The model under review builds one solid part; all positions refer to its coordinate system, in mm. Round coordinates to 2 decimals unless told otherwise and drop trailing zeros. Order: outer loops, then holes, each group sorted by start corner. A loop starts at its lowest first (then second) coordinate and runs counter-clockwise, first axis right, second up. Notation, with made-up numbers: (38, -6.5) -> (85, -6.5) arc R18 cw to (85, 21.5) -> close; hole circle Ø1 at (61, -32). An arc over 180 degrees is marked (long way). Return JSON: item names as keys, results as strings. Group by question number.
from build123d import *

# Parameters (mm, degrees)
BOSS_EXTRUDE1_DEPTH = 6.35
SKETCH2_R           = 12.5
CUT_EXTRUDE1_DEPTH  = 414.4708728


with BuildPart() as part:
    # Sketch1 → Boss-Extrude1 (new body)
    with BuildSketch(Plane.XY):
        Polygon((-381.094249826, -159.734501203), (-381.094249826, 25), (380.905750174, 25), (380.905750174, -160.265445134), align=None)
    extrude(amount=BOSS_EXTRUDE1_DEPTH)

    # Sketch2 → Cut-Extrude1 (cut, through all)
    with BuildSketch(Plane.XY.offset(6.35)):
        Circle(SKETCH2_R)
    extrude(amount=-CUT_EXTRUDE1_DEPTH, mode=Mode.SUBTRACT)


solid = part.part
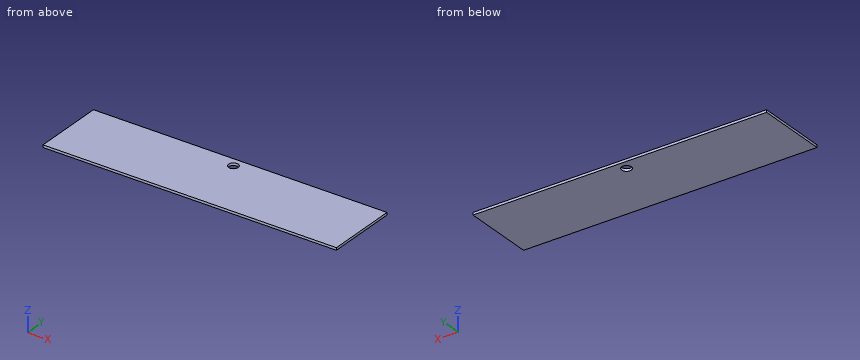
Item 1: Insertion check: pin 1 Ø3 at (x, z) = (264, 4) entering from -Y; pin 2 Ø1.5 at (x, z) = (-146.5, 1) entering from -Y. Each pin has a flat end and moves straight along its axis. Give the tip position at first contact, or say it passes through.
Item 2: Consider section B-B on y = 0. State the section outline as (x, z) points.
Item 3: Wall thickness on line 1 along Y through (x, z) = (237, 2.75); line 2 along Y through (x, z) = (-193.5, 0.5); line 3 along Y through (x, z) = (0, 1.5): over which ranges is each line inside the solid? List them lowest first.
Item 4: Consider section A-A on x = -3. State the section outline as (y, z) points.
Values:
{
 "1": {"pin 1": "y = -160.19", "pin 2": "y = -159.9"},
 "2": {"outline": "(-381.09, 0) -> (-12.5, 0) -> (-12.5, 6.35) -> (-381.09, 6.35) -> close; (12.5, 0) -> (380.91, 0) -> (380.91, 6.35) -> (12.5, 6.35) -> close"},
 "3": {"line 1": "-160.17 to 25", "line 2": "-159.87 to 25", "line 3": "-160 to -12.5, 12.5 to 25"},
 "4": {"outline": "(-160, 0) -> (-12.13, 0) -> (-12.13, 6.35) -> (-160, 6.35) -> close; (12.13, 0) -> (25, 0) -> (25, 6.35) -> (12.13, 6.35) -> close"}
}
